```python
from build123d import *

# Parameters (mm, degrees)
SKETCH1_W           = 61.5
SKETCH1_H           = 43
BOSS_EXTRUDE1_DEPTH = 2
SKETCH2_W           = 89
SKETCH2_H           = 54
BOSS_EXTRUDE2_DEPTH = 3
CUT_EXTRUDE1_REACH  = 114.472
SKETCH3_R           = 1.5
CUT_EXTRUDE2_REACH  = 113.136


with BuildPart() as part:
    # Sketch1 → Boss-Extrude1 (new body)
    with BuildSketch(Plane.XY):
        with BuildLine():
            Line((2, 0), (93, 0))
            ThreePointArc((93, 0), (94.414213562, 0.585786438), (95, 2))
            Line((95, 2), (95, 58))
            ThreePointArc((95, 58), (94.414213562, 59.414213562), (93, 60))
            Line((93, 60), (2, 60))
            ThreePointArc((2, 60), (0.585786438, 59.414213562), (0, 58))
            Line((0, 58), (0, 2))
            ThreePointArc((0, 2), (0.585786438, 0.585786438), (2, 0))
        make_face()
        with Locations((41.25, 29.5)):
            Rectangle(SKETCH1_W, SKETCH1_H, mode=Mode.SUBTRACT)
    extrude(amount=BOSS_EXTRUDE1_DEPTH)

    # Sketch2 → Boss-Extrude2 (add)
    with BuildSketch(Plane(origin=(0, 0, 0), x_dir=(-1, 0, 0), z_dir=(0, 0, -1))):
        with BuildLine():
            Line((-93.5, 58), (-93.5, 2))
            ThreePointArc((-93.5, 2), (-93.353553391, 1.646446609), (-93, 1.5))
            Line((-93, 1.5), (-2, 1.5))
            ThreePointArc((-2, 1.5), (-1.646446609, 1.646446609), (-1.5, 2))
            Line((-1.5, 2), (-1.5, 58))
            ThreePointArc((-1.5, 58), (-1.646446609, 58.353553391), (-2, 58.5))
            Line((-2, 58.5), (-93, 58.5))
            ThreePointArc((-93, 58.5), (-93.353553391, 58.353553391), (-93.5, 58))
        make_face()
        with Locations((-47.5, 30)):
            Rectangle(SKETCH2_W, SKETCH2_H, mode=Mode.SUBTRACT)
    extrude(amount=BOSS_EXTRUDE2_DEPTH)

    # Sketch3 → Cut-Extrude1 (cut, up to next)
    with BuildSketch(Plane.XY.offset(2), mode=Mode.PRIVATE) as cut_extrude1_sk1:
        with Locations((7.75, 48)):
            Circle(SKETCH3_R)
    cut_extrude1_tool1 = extrude(cut_extrude1_sk1.sketch, amount=-CUT_EXTRUDE1_REACH, mode=Mode.PRIVATE) & part.part
    # Sketch3 → Cut-Extrude1 (cut, up to next)
    with BuildSketch(Plane.XY.offset(2), mode=Mode.PRIVATE) as cut_extrude1_sk2:
        with Locations((74.75, 48)):
            Circle(SKETCH3_R)
    cut_extrude1_tool2 = extrude(cut_extrude1_sk2.sketch, amount=-CUT_EXTRUDE1_REACH, mode=Mode.PRIVATE) & part.part
    # Sketch3 → Cut-Extrude1 (cut, up to next)
    with BuildSketch(Plane.XY.offset(2), mode=Mode.PRIVATE) as cut_extrude1_sk3:
        with Locations((7.75, 11)):
            Circle(SKETCH3_R)
    cut_extrude1_tool3 = extrude(cut_extrude1_sk3.sketch, amount=-CUT_EXTRUDE1_REACH, mode=Mode.PRIVATE) & part.part
    # Sketch3 → Cut-Extrude1 (cut, up to next)
    with BuildSketch(Plane.XY.offset(2), mode=Mode.PRIVATE) as cut_extrude1_sk4:
        with Locations((74.75, 11)):
            Circle(SKETCH3_R)
    cut_extrude1_tool4 = extrude(cut_extrude1_sk4.sketch, amount=-CUT_EXTRUDE1_REACH, mode=Mode.PRIVATE) & part.part
    add(cut_extrude1_tool1.solids().sort_by_distance((7.75, 48, 2))[0], mode=Mode.SUBTRACT)
    add(cut_extrude1_tool2.solids().sort_by_distance((74.75, 48, 2))[0], mode=Mode.SUBTRACT)
    add(cut_extrude1_tool3.solids().sort_by_distance((7.75, 11, 2))[0], mode=Mode.SUBTRACT)
    add(cut_extrude1_tool4.solids().sort_by_distance((74.75, 11, 2))[0], mode=Mode.SUBTRACT)

    # Sketch4 → Cut-Extrude2 (cut, up to next)
    with BuildSketch(Plane(origin=(93.5, 0, 0), x_dir=(0, 0, -1), z_dir=(1, 0, 0)), mode=Mode.PRIVATE) as cut_extrude2_sk1:
        with BuildLine():
            Line((6.35854024, 11.62115589), (3.091503029, 11.62115589))
            ThreePointArc((3.091503029, 11.62115589), (1.677289466, 12.206942328), (1.091503029, 13.62115589))
            Line((1.091503029, 13.62115589), (1.091503029, 50.941867475))
            ThreePointArc((1.091503029, 50.941867475), (1.677289466, 52.356081037), (3.091503029, 52.941867475))
            Line((3.091503029, 52.941867475), (6.35854024, 52.941867475))
            ThreePointArc((6.35854024, 52.941867475), (7.772753802, 52.356081037), (8.35854024, 50.941867475))
            Line((8.35854024, 50.941867475), (8.35854024, 13.62115589))
            ThreePointArc((8.35854024, 13.62115589), (7.772753802, 12.206942328), (6.35854024, 11.62115589))
        make_face()
    cut_extrude2_tool1 = extrude(cut_extrude2_sk1.sketch, amount=-CUT_EXTRUDE2_REACH, mode=Mode.PRIVATE) & part.part
    add(cut_extrude2_tool1.solids().sort_by_distance((93.5, 32.281512, -4.725022))[0], mode=Mode.SUBTRACT)


solid = part.part
```
Build history of the part. All positions in model axes, mm. A direction names the side the tool comes from. Give positions to 0.01 mm unless a question says otherwise; leave off trailing zeros. Loops run counter-clockwise (first coordinate to the right, second up) from the corner with the lowest first, then second, coordinate; pieces in that order, holes last.
Item 1: Slice it at A-A, the plane x = 16. List the corners of the cut face in (y, z), and give its area (3 significant figures).
Answers follow:
outline: (0, 0) - (1.5, 0) - (1.5, -3) - (3, -3) - (3, 0) - (8, 0) - (8, 2) - (0, 2) - close; (51, 0) - (57, 0) - (57, -3) - (58.5, -3) - (58.5, 0) - (60, 0) - (60, 2) - (51, 2) - close
area: 43.0 mm2
Item 2: Pull direction Y, two halves, no side cores. Call faces 6 (the face through (94.43, 59.4, 0.99)), 7 (the face through (51.1, 2.7, -3)), 8 (the face through (10.5, 29, 1)), 9 (the face through (7.425, 46.536, 1.014)): released by +Y, released by -Y, zero draft, split by the parting line, or undercut.
Answers follow:
face 6: released by +Y
face 7: zero draft
face 8: undercut
face 9: undercut
Item 3: Drill centre lines: line 1 (Y direction, x = 74.75, z = 1); line 2 (Y direction, x = 32.5, z = -2.2); line 3 (X direction, y = 37, z = -0.8). Where is each one in solid material? Low to high.
Answers follow:
line 1: y = 0 to 9.5, 12.5 to 46.5, 49.5 to 60
line 2: y = 1.5 to 3, 57 to 58.5
line 3: x = 1.5 to 3, 92 to 93.5
Item 4: Flat gauge pins, fed straight in: pin 1 (3.5 mm diameter, centred on x = 74.75, y = 11, fed in from +Z); pin 2 (0.9 mm diameter, centred on x = 49, z = -1.5, fed in from +Y); pin 3 (2.5 mm diameter, centred on x = 7.75, y = 11, fed in from +Z); pin 4 (0.9 mm diameter, centred on y = 30.5, z = -1, fed in from -X). Where does each tip first touch, or does it go through?
Answers follow:
pin 1: stops at z = 2
pin 2: stops at y = 58.5
pin 3: passes through
pin 4: stops at x = 1.5
Item 5: Slice it at C-C, the plane x = 89.5. List the corners of the cut face in (y, z), and give its area (3 significant figures).
Answers follow:
outline: (0, 0) - (1.5, 0) - (1.5, -3) - (3, -3) - (3, 0) - (57, 0) - (57, -3) - (58.5, -3) - (58.5, 0) - (60, 0) - (60, 2) - (0, 2) - close
area: 129 mm2
Item 6: Which spindle directions (+Z, -Z, +X, -X, +Y, -Y) get a long thin tool onto all of the face, cutting with end or side? Do faces 1 (the face through (72, 29, 1)), 2 (the face through (92.76, 12.224, -1.66)), 3 (the face through (47, 58.5, -1)), 4 (the face through (92, 29.6, -0.8)), 5 (the face through (1.5, 30, -1)). Say none if no direction does.
Answers follow:
face 1: +Z, -Z
face 2: -Z, +X
face 3: -Z, +X, -X, +Y
face 4: -Z
face 5: -Z, -X, +Y, -Y
Item 7: Slice it at B-B, the plane y = 34. List the corners of the cut face in (x, z), and give its area (3 significant figures).
Answers follow:
outline: (0, 0) - (1.5, 0) - (1.5, -3) - (3, -3) - (3, 0) - (10.5, 0) - (10.5, 2) - (0, 2) - close; (72, 0) - (92, 0) - (92, -1.09) - (93.5, -1.09) - (93.5, 0) - (95, 0) - (95, 2) - (72, 2) - close
area: 73.1 mm2
Item 8: Slice it at D-D, the plane y = 48. List the corners of the cut face in (x, z), and give its area (3 significant figures).
Answers follow:
outline: (0, 0) - (1.5, 0) - (1.5, -3) - (3, -3) - (3, 0) - (6.25, 0) - (6.25, 2) - (0, 2) - close; (9.25, 0) - (10.5, 0) - (10.5, 2) - (9.25, 2) - close; (72, 0) - (73.25, 0) - (73.25, 2) - (72, 2) - close; (76.25, 0) - (92, 0) - (92, -1.09) - (93.5, -1.09) - (93.5, 0) - (95, 0) - (95, 2) - (76.25, 2) - close
area: 61.1 mm2
